Model file for the job. Use its own axes, mm. Round coordinates to 2 decimals unless told otherwise and drop trailing zeros. Loops run counter-clockwise (first coordinate to the right, second up) from the corner with the lowest first, then second, coordinate; pieces in that order, holes last. Notation, with made-up numbers: (49.5, 38.25) -> (97.5, 38.25) arc R24 ccw to (97.5, 73.25) -> close; hole circle Ø8 at (-7, -24). An arc over 180 degrees is marked (long way). Use a Markdown table: item, result. Add a question column.
```python
from build123d import *

# Parameters (mm, degrees)
F0_W     = 100
F0_H     = 50
F1_DEPTH = 12.5
F2_SIZE  = 25.7
F3_R     = 0.2


with BuildPart() as f1:
    # F0 (on Top) → F1 (new body)
    with BuildSketch(Plane.XY):
        with Locations((50, 25)):
            Rectangle(F0_W, F0_H)
    extrude(amount=-F1_DEPTH)

    # F2
    f2_edges = [f1.edges().sort_by_distance(p)[0] for p in [
        (100, 50, -6.25),
    ]]
    chamfer(f2_edges, length=F2_SIZE)

    # F3
    f3_edges = [f1.edges().sort_by_distance(p)[0] for p in [
        (100, 12.15, 0),
        (87.15, 37.15, 0),
        (50, 0, 0),
        (37.15, 50, 0),
        (0, 25, 0),
        (100, 12.15, -12.5),
        (87.15, 37.15, -12.5),
        (50, 0, -12.5),
        (37.15, 50, -12.5),
        (0, 25, -12.5),
    ]]
    fillet(f3_edges, radius=F3_R)


solid = f1.part
```
1) Pin check, flat tip, straight feed: pin 1 Ø3 at (x, z) = (89, -5) entering from +Y. Stop position of the tip, or through.
2) Wall check: probe 1 along Y at (x, z) = (74.5, -2); probe 2 along X at (y, z) = (38, -6.75); probe 3 along X at (y, z) = (32.5, -5). Give the ranges that are in metal, low to high. Write a range as from..to.
3) Cut at A-A on z = -10.5. Write the cut outline in (x, y).
Established:
| question | item | result |
|---|---|---|
| 1 | pin 1 | stops at y = 36.8 |
| 2 | probe 1 | y = 0..49.8 |
| 2 | probe 2 | x = 0..86.3 |
| 2 | probe 3 | x = 0..91.8 |
| 3 | outline | (0, 0) -> (100, 0) -> (100, 24.3) -> (74.3, 50) -> (0, 50) -> close |
